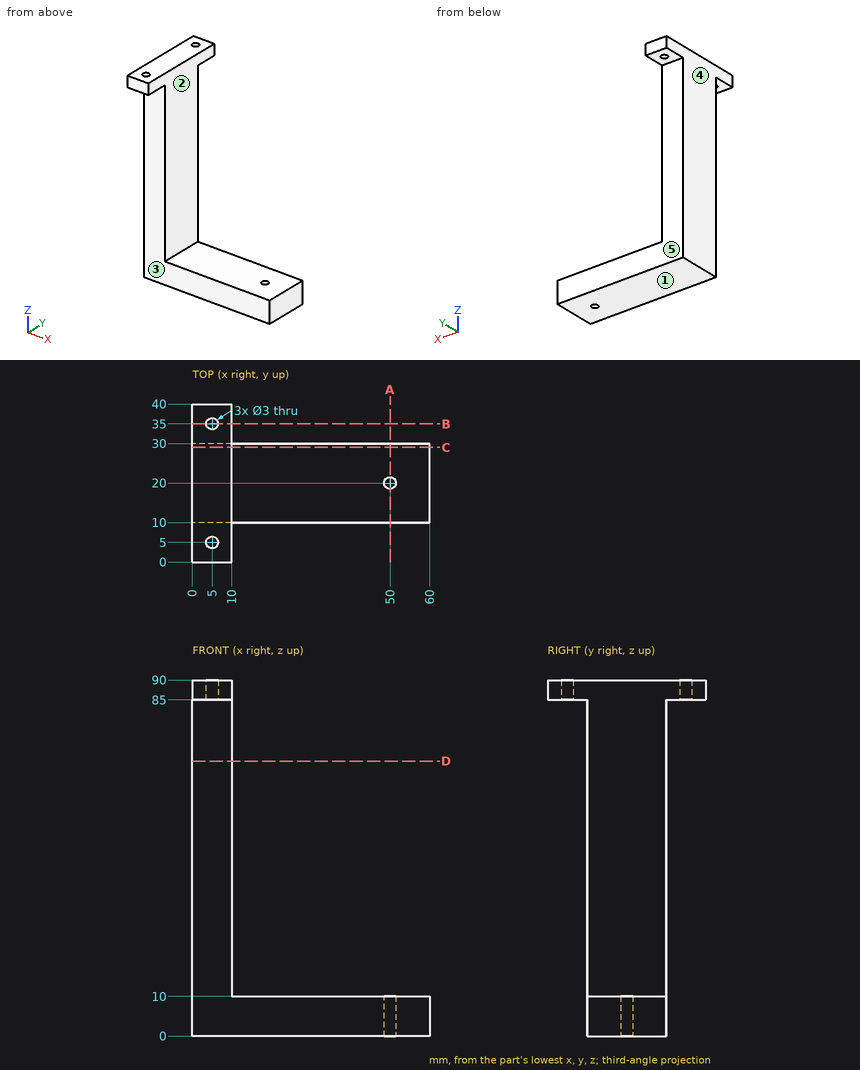
Study the drawing (mm; zero at the part's minimum x, y, z) and answer. A direction names the side the tool comes from. Give positions to 0.01 mm unless a question says otherwise; leave off trailing zeros. Loops run counter-clockwise (first coordinate to the right, second up) from the corner with the lowest first, then second, coordinate; pieces in that order, holes last. Notation, with made-up numbers: (13, 65.5) - (48, 65.5) arc R27 cw to (48, 100.5) - close; hole circle Ø2 at (-23.5, 83). An arc over 180 degrees is marked (long way). Answer as CSV lines item,"result". Start each with the question number.
1) Each of these flat-tipped pins is pushed along its axis until it touches: pin 1 Ø3.5 at (x, y) = (50, 20) entering from +Z; pin 2 Ø3 at (x, y) = (7, 7) entering from -Z; pin 3 Ø10 at (y, z) = (14, 15) entering from -X; pin 4 Ø12 at (y, z) = (26, 45.5) entering from +X. Where does it stop, or does it pass through?
2) Straight lines are drawn through the part: L1, parallel to Y at x = 5, z = 87; L2, parallel to Z at x = 13, y = 11.5. For each, find the intervals that lie inside material, in ascending order. Write a range as from..to.
3) Which of the six approach directions +Z, -Z, +X, -X, +Y, -Y give full straight-line access (tool end or side, diameter ignored) to the marked faces 1, 2, 3, 4 and 5?
4) Find section C-C (y = 29). Write down the section's boundary in (x, z).
5) Find section D-D (z = 69.5). Write down the section's boundary in (x, y).
6) Find section A-A (x = 50). Write down the section's boundary in (y, z).
7) Find section B-B (y = 35). Write down the section's boundary in (x, z), then the cut area to 3 significant figures.
Findings below:
1,pin 1,"z = 10"
1,pin 2,"z = 85"
1,pin 3,"x = 0"
1,pin 4,"x = 10"
2,L1,"0..3.5, 6.5..33.5, 36.5..40"
2,L2,"0..10"
3,face 1,"-Z, +X, -X, +Y, -Y"
3,face 2,"+Z, +X, +Y, -Y"
3,face 3,"-Z, +X, -X, -Y"
3,face 4,"+Z, -Z, -X, +Y, -Y"
3,face 5,"-Z, +X, -X, +Y"
4,outline,"(0, 0) - (60, 0) - (60, 10) - (10, 10) - (10, 90) - (0, 90) - close"
5,outline,"(0, 10) - (10, 10) - (10, 30) - (0, 30) - close"
6,outline,"(10, 0) - (18.5, 0) - (18.5, 10) - (10, 10) - close; (21.5, 0) - (30, 0) - (30, 10) - (21.5, 10) - close"
7,outline,"(0, 85) - (3.5, 85) - (3.5, 90) - (0, 90) - close; (6.5, 85) - (10, 85) - (10, 90) - (6.5, 90) - close"
7,area,"35.0 mm^2"
